Could you check a few things on this model? Use its own coordinates, in mm. Face numbers are marked on the shaded views. Round coordinates to 2 decimals unless told otherwise and drop trailing zeros. Write each loop counter-clockwise with the first axis right and the second up, starting at its lowest first coordinate (ties: lowest second). Pieces come first, ordered by that corner, then holes. Notation, with made-up numbers: (14, -37) -> (69, -37) arc R7 ccw to (69, -30) -> close; hole circle Ø7 at (59, 42.25). An arc over 180 degrees is marked (long way). Answer in a Markdown table with one row per item.
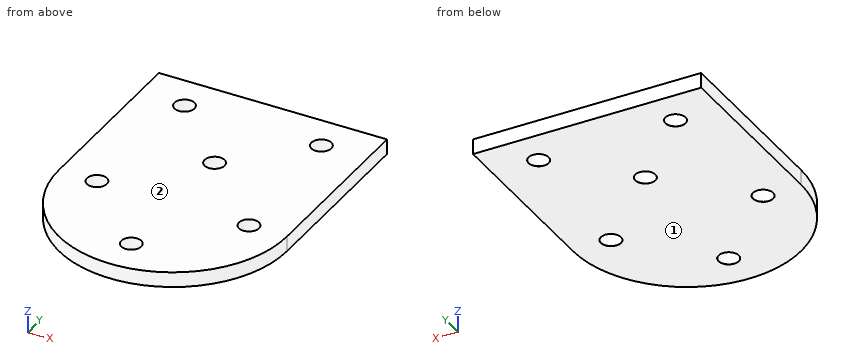
from build123d import *

# Parameters (mm, degrees)
BOSS_EXTRUDE1_DEPTH            = 5
M6_CLEARANCE_HOLE2_D           = 6.6
M6_CLEARANCE_HOLE2_CSINK_D     = 6.65
M6_CLEARANCE_HOLE2_CSINK_ANGLE = 90


with BuildPart() as part:
    # Sketch6 → Boss-Extrude1 (new body)
    with BuildSketch(Plane.XY):
        with BuildLine():
            Line((37.5, 0), (37.5, 60))
            Line((37.5, 60), (-37.5, 60))
            Line((-37.5, 60), (-37.5, 0))
            ThreePointArc((-37.5, 0), (0, -37.5), (37.5, 0))
        make_face()
    extrude(amount=BOSS_EXTRUDE1_DEPTH)

    # M6 Clearance Hole2 (through all)
    with Locations(Plane(origin=(0, 0, 0), x_dir=(-1, 0, 0), z_dir=(0, 0, -1))):
        with Locations((-22.5, 48), (22.5, 48), (0, 25), (25, 0), (0, -25), (-25, 0)):
            CounterSinkHole(M6_CLEARANCE_HOLE2_D / 2, M6_CLEARANCE_HOLE2_CSINK_D / 2, counter_sink_angle=M6_CLEARANCE_HOLE2_CSINK_ANGLE)


solid = part.part
1) For pin 1 (4 mm diameter, centred on x = 22.5, y = 48, fed in from -Z) (1 decimal), with a flat end and sliding along its axis, tell me the tip position at first contact or that it passes through.
Findings:
| item | result |
|---|---|
| pin 1 | passes through |
2) Imagine slicing it at B-B, the plane x = 0. Please give me the cut outline in (y, z) (3 decimals), plus the area to 4 significant figures.
Findings:
| item | result |
|---|---|
| outline | (-37.5, 0) -> (-28.325, 0) -> (-28.3, 0.025) -> (-28.3, 5) -> (-37.5, 5) -> close; (-21.7, 0.025) -> (-21.675, 0) -> (21.675, 0) -> (21.7, 0.025) -> (21.7, 5) -> (-21.7, 5) -> close; (28.3, 0.025) -> (28.325, 0) -> (60, 0) -> (60, 5) -> (28.3, 5) -> close |
| area | 421.5 mm^2 |
3) Imagine slicing it at C-C, the plane z = 2.75. Please give me the cut outline in (x, y).
Findings:
| item | result |
|---|---|
| outline | (-37.5, 0) arc R37.5 ccw to (37.5, 0) -> (37.5, 60) -> (-37.5, 60) -> close; hole circle Ø6.6 at (-25, 0); hole circle Ø6.6 at (-22.5, 48); hole circle Ø6.6 at (0, -25); hole circle Ø6.6 at (0, 25); hole circle Ø6.6 at (22.5, 48); hole circle Ø6.6 at (25, 0) |
4) Imagine slicing it at D-D, the plane y = 48. Please give me the cut outline in (x, z) (3 decimals).
Findings:
| item | result |
|---|---|
| outline | (-37.5, 0) -> (-25.825, 0) -> (-25.8, 0.025) -> (-25.8, 5) -> (-37.5, 5) -> close; (-19.2, 0.025) -> (-19.175, 0) -> (19.175, 0) -> (19.2, 0.025) -> (19.2, 5) -> (-19.2, 5) -> close; (25.8, 0.025) -> (25.825, 0) -> (37.5, 0) -> (37.5, 5) -> (25.8, 5) -> close |
5) Please list where these lines run through material, in increasing order: line 1 (Y direction, x = 0, z = 3.65); line 2 (X direction, y = 48, z = 1.35); line 3 (X direction, y = 0, z = 3.2).
Findings:
| item | result |
|---|---|
| line 1 | y = -37.5 to -28.3, -21.7 to 21.7, 28.3 to 60 |
| line 2 | x = -37.5 to -25.8, -19.2 to 19.2, 25.8 to 37.5 |
| line 3 | x = -37.5 to -28.3, -21.7 to 21.7, 28.3 to 37.5 |
6) Thinking about a two-plate mould opening in Z: for the marked faces 1 and 2, which applies, +Z half, -Z half, draft (parallel to the pull), parting line (faces both ways), or undercut?
Findings:
| item | result |
|---|---|
| face 1 | -Z half |
| face 2 | +Z half |
7) Imagine slicing it at A-A, the plane y = 25. Please give me the cut outline in (x, z) (3 decimals).
Findings:
| item | result |
|---|---|
| outline | (-37.5, 0) -> (-3.325, 0) -> (-3.3, 0.025) -> (-3.3, 5) -> (-37.5, 5) -> close; (3.3, 0.025) -> (3.325, 0) -> (37.5, 0) -> (37.5, 5) -> (3.3, 5) -> close |
